Geometry check sheet. Reference: drawing and pictorial views, mm from the part's lowest x, y, z. A direction names the side the tool comes from. Give positions to 0.01 mm unless a question says otherwise; leave off trailing zeros. Write each loop counter-clockwise with the first axis right and the second up, starting at its lowest first coordinate (ties: lowest second). Pieces come first, ordered by that corner, then holes.
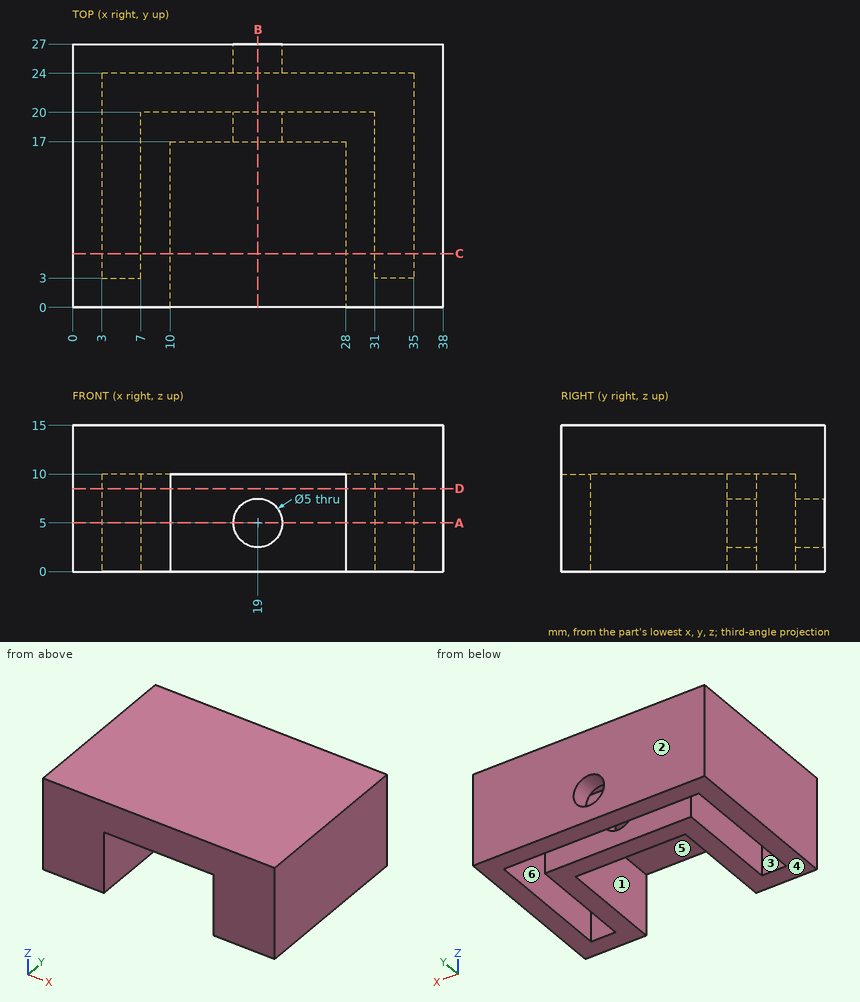
Item 1: Sectioned sample at A-A on z = 5. Record the cut outline in (x, y), then the cut area to 3 significant figures.
Answer key:
outline: (0, 0) - (10, 0) - (10, 17) - (16.5, 17) - (16.5, 20) - (7, 20) - (7, 3) - (3, 3) - (3, 24) - (16.5, 24) - (16.5, 27) - (0, 27) - close; (21.5, 17) - (28, 17) - (28, 0) - (38, 0) - (38, 27) - (21.5, 27) - (21.5, 24) - (35, 24) - (35, 3) - (31, 3) - (31, 20) - (21.5, 20) - close
area: 426 mm2
Item 2: Sectioned sample at B-B on x = 19. Record the cut outline in (y, z).
Answer key:
outline: (0, 10) - (17, 10) - (17, 7.5) - (20, 7.5) - (20, 10) - (24, 10) - (24, 7.5) - (27, 7.5) - (27, 15) - (0, 15) - close; (17, 0) - (20, 0) - (20, 2.5) - (17, 2.5) - close; (24, 0) - (27, 0) - (27, 2.5) - (24, 2.5) - close
Item 3: Release check for a two-part mould opening along Y. For the marked faces 1, 2 and 3 record: released by +Y, released by -Y, zero draft, split by the parting line, or undercut.
Answer key:
face 1: zero draft
face 2: released by +Y
face 3: undercut
Item 4: Set-up check for the marked faces 4, 5 and 6: record each of +Z, -Z, +X, -X, +Y, -Y from which the full face is reachable in a straight line by a thin tool's end or side.
Answer key:
face 4: -Z, +X, -X, +Y, -Y
face 5: -Z, -Y
face 6: -Z
Item 5: Sectioned sample at D-D on z = 8.5. Record the cut outline in (x, y), then the cut area to 3 significant figures.
Answer key:
outline: (0, 0) - (10, 0) - (10, 17) - (28, 17) - (28, 0) - (38, 0) - (38, 27) - (0, 27) - close; hole (3, 3) - (7, 3) - (7, 20) - (31, 20) - (31, 3) - (35, 3) - (35, 24) - (3, 24) - close
area: 456 mm2
Item 6: Depth check by flat-ended pin: pin 1 (3 mm diameter, centred on y = 15, z = 12.5, fed in from -X); pin 2 (5 mm diameter, centred on x = 18.5, z = 3, fed in from -Y). Enter the tip coordinate at first touch or a pass-through.
Answer key:
pin 1: stops at x = 0
pin 2: stops at y = 17
Item 7: Sectioned sample at C-C on y = 5.5. Record the cut outline in (x, z), then the cut area to 3 significant figures.
Answer key:
outline: (0, 0) - (3, 0) - (3, 10) - (7, 10) - (7, 0) - (10, 0) - (10, 10) - (28, 10) - (28, 0) - (31, 0) - (31, 10) - (35, 10) - (35, 0) - (38, 0) - (38, 15) - (0, 15) - close
area: 310 mm2
Item 8: Scan lines: line 1 along X through (y, z) = (19.4, 5); line 2 along X through (y, z) = (16, 8); line 3 along Z through (x, y) = (19, 17.95). Record each from-to range of solid material in increasing order.
Answer key:
line 1: x = 0 to 3, 7 to 16.5, 21.5 to 31, 35 to 38
line 2: x = 0 to 3, 7 to 10, 28 to 31, 35 to 38
line 3: z = 0 to 2.5, 7.5 to 15
